Could you check a few things on this drawing? It's one solid part, dimensions in mm from its lowest x, y, z. Round coordinates to 2 decimals unless told otherwise and drop trailing zeros. Loops run counter-clockwise (first coordinate to the right, second up) from the corner with the lowest first, then second, coordinate; pieces in that order, holes last. Notation, with made-up numbers: (67.25, 56.25) -> (119.25, 56.25) arc R28 ccw to (119.25, 81.25) -> close; hole circle Ø9 at (5.5, 78.25). An arc over 180 degrees is marked (long way). Put each result on its own line as item: value. Start each with the question number.
1. I'm going to push a flat-ended pin straight in: P1, Ø11, axis at x = 218, y = 410.5, coming from the -Z side. Where does the tip first touch, or does it pass through?
2. Imagine slicing it at A-A, the plane y = 29.5. Please give me the cut outline in (x, z) (1 decimal), and give its area (3 significant figures).
3. I need wall thicknesses on line 1 (X direction, y = 41, z = 2) (1 decimal); line 2 (Y direction, x = 233.5, z = 11.25); line 3 (Y direction, x = 213.5, z = 6) (1 decimal). Which ranges of each line are inside material? Lowest first, please. Write a range as [from, to].
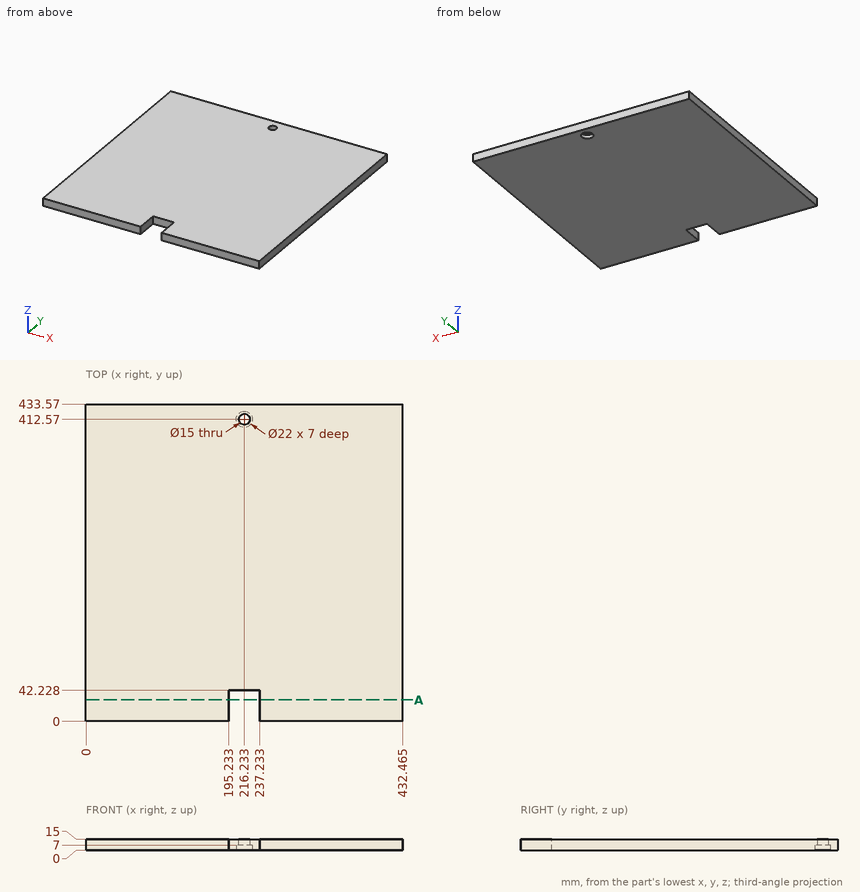
Entries:
1. P1: z = 7
2. outline: (0, 0) -> (195.2, 0) -> (195.2, 15) -> (0, 15) -> close; (237.2, 0) -> (432.5, 0) -> (432.5, 15) -> (237.2, 15) -> close
2. area: 5,860 mm^2
3. line 1: [0, 195.2], [237.2, 432.5]
3. line 2: [42.23, 433.57]
3. line 3: [42.2, 401.9], [423.2, 433.6]
